from build123d import *

# Parameters (mm, degrees)
SKETCH1_W               = 40.35
SKETCH1_H               = 43.35
BOSS_EXTRUDE1_DEPTH     = 47
CUT_EXTRUDE2_DEPTH      = 102
FILLET1_R               = 10
CUT_EXTRUDE3_DEPTH      = 102
FILLET2_R               = 5
SKETCH6_R               = 1.73
CUT_EXTRUDE4_DEPTH      = 102
CUT_EXTRUDE4_DEPTH_BACK = 102
CUT_EXTRUDE5_DEPTH      = 102
SKETCH8_R               = 1.55
CUT_EXTRUDE6_DEPTH      = 102


with BuildPart() as part:
    # Sketch1 → Boss-Extrude1 (new body)
    with BuildSketch(Plane(origin=(0, 0, 0), x_dir=(1, 0, 0), z_dir=(0, 1, 0))):
        with Locations((-26.966212793, -29.108023223)):
            Rectangle(SKETCH1_W, SKETCH1_H)
    extrude(amount=BOSS_EXTRUDE1_DEPTH)

    # Sketch3 → Cut-Extrude2 (cut)
    with BuildSketch(Plane.XY.offset(50.783023223)):
        with BuildLine():
            Line((-47.141212793, 47), (-47.141212793, 26.825))
            ThreePointArc((-47.141212793, 26.825), (-41.232092103, 41.09087931), (-26.966212793, 47))
            Line((-26.966212793, 47), (-47.141212793, 47))
        make_face()
        with BuildLine():
            Line((-6.791212793, 47), (-26.966212793, 47))
            ThreePointArc((-26.966212793, 47), (-12.700333482, 41.09087931), (-6.791212793, 26.825))
            Line((-6.791212793, 26.825), (-6.791212793, 47))
        make_face()
    extrude(amount=-CUT_EXTRUDE2_DEPTH, mode=Mode.SUBTRACT)

    # Fillet1
    fillet1_edges = [part.edges().sort_by_distance(p)[0] for p in [
        (-26.966212793, 0, 50.783023223),
    ]]
    fillet(fillet1_edges, radius=FILLET1_R)

    # Sketch5 → Cut-Extrude3 (cut)
    with BuildSketch(Plane.ZY.offset(47.141212793)):
        with BuildLine():
            Line((-6.665763497, 3.45), (36.595559978, 3.45))
            Line((36.595559978, 3.45), (40.783023223, 3.45))
            ThreePointArc((40.783023223, 3.45), (45.41457264, 5.368450583), (47.333023223, 10))
            Line((47.333023223, 10), (47.333023223, 17.578484004))
            Line((47.333023223, 17.578484004), (47.333023223, 59.778436909))
            Line((47.333023223, 59.778436909), (-6.665763497, 59.778436909))
            Line((-6.665763497, 59.778436909), (-6.665763497, 3.45))
        make_face()
    extrude(amount=-CUT_EXTRUDE3_DEPTH, mode=Mode.SUBTRACT)

    # Fillet2
    fillet2_edges = [part.edges().sort_by_distance(p)[0] for p in [
        (-6.791212793, 1.725, 7.433023223),
        (-47.141212793, 1.725, 7.433023223),
    ]]
    fillet(fillet2_edges, radius=FILLET2_R)

    # Sketch6 → Cut-Extrude4 (cut, two sides)
    with BuildSketch(Plane(origin=(0, 3.45, 0), x_dir=(1, 0, 0), z_dir=(0, 1, 0))) as cut_extrude4_sk:
        with BuildLine():
            Line((-10.653989329, -40.783023223), (-13.388436256, -40.783023223))
            ThreePointArc((-13.388436256, -40.783023223), (-12.021212793, -41.453023223), (-10.653989329, -40.783023223))
        make_face()
        with BuildLine():
            ThreePointArc((-12.021212793, -37.993023223), (-13.57470885, -38.961741409), (-13.388436256, -40.783023223))
            Line((-13.388436256, -40.783023223), (-10.653989329, -40.783023223))
            ThreePointArc((-10.653989329, -40.783023223), (-10.384417663, -40.283203287), (-10.291212793, -39.723023223))
            ThreePointArc((-10.291212793, -39.723023223), (-10.797918061, -38.499728491), (-12.021212793, -37.993023223))
        make_face()
        with BuildLine():
            ThreePointArc((-41.911212793, -37.993023223), (-43.134507524, -38.499728491), (-43.641212793, -39.723023223))
            ThreePointArc((-43.641212793, -39.723023223), (-43.548007922, -40.283203287), (-43.278436256, -40.783023223))
            Line((-43.278436256, -40.783023223), (-40.543989329, -40.783023223))
            ThreePointArc((-40.543989329, -40.783023223), (-40.274417663, -40.283203287), (-40.181212793, -39.723023223))
            ThreePointArc((-40.181212793, -39.723023223), (-40.687918061, -38.499728491), (-41.911212793, -37.993023223))
        make_face()
        with BuildLine():
            Line((-40.543989329, -40.783023223), (-43.278436256, -40.783023223))
            ThreePointArc((-43.278436256, -40.783023223), (-41.911212793, -41.453023223), (-40.543989329, -40.783023223))
        make_face()
        with Locations((-12.021212793, -15.663023223)):
            Circle(SKETCH6_R)
        with Locations((-41.911212793, -15.663023223)):
            Circle(SKETCH6_R)
    extrude(amount=CUT_EXTRUDE4_DEPTH, mode=Mode.SUBTRACT)
    extrude(cut_extrude4_sk.sketch, amount=-CUT_EXTRUDE4_DEPTH_BACK, mode=Mode.SUBTRACT)

    # Sketch7 → Cut-Extrude5 (cut)
    with BuildSketch(Plane.XY.offset(50.783023223)):
        with BuildLine():
            Line((-33.541212793, 33.925), (-33.541212793, 19.945))
            ThreePointArc((-33.541212793, 19.945), (-26.966212793, 13.37), (-20.391212793, 19.945))
            Line((-20.391212793, 19.945), (-20.391212793, 33.925))
            ThreePointArc((-20.391212793, 33.925), (-26.966212793, 40.5), (-33.541212793, 33.925))
        make_face()
    extrude(amount=-CUT_EXTRUDE5_DEPTH, mode=Mode.SUBTRACT)

    # Sketch8 → Cut-Extrude6 (cut)
    with BuildSketch(Plane.XY.offset(50.783023223)):
        with Locations((-42.516212793, 26.825)):
            Circle(SKETCH8_R)
        with Locations((-34.766212793, 40.277230298)):
            Circle(SKETCH8_R)
        with Locations((-34.766212793, 13.372769702)):
            Circle(SKETCH8_R)
        with Locations((-19.166212793, 13.372769702)):
            Circle(SKETCH8_R)
        with Locations((-11.416212793, 26.825)):
            Circle(SKETCH8_R)
        with Locations((-19.166212793, 40.277230298)):
            Circle(SKETCH8_R)
    extrude(amount=-CUT_EXTRUDE6_DEPTH, mode=Mode.SUBTRACT)


solid = part.part
Build history of the part. All positions in model axes, mm. A direction names the side the tool comes from. Coordinates: 2 decimals unless noted, no trailing zeros. Order: outer loops, then holes, each group sorted by start corner. A loop starts at its lowest first (then second) coordinate and runs counter-clockwise, first axis right, second up. Notation, with made-up numbers: M 10.25,-37 L 57.25,-37 A15 ccw 57.25,-17 Z; hole C 36,77 d4. An arc over 180 degrees is marked long. One line per question, with ' | ' between items. Start each with the question number.
Q1. Saw through at A-A (y = 37). List the corners of the cut face in (x, z), then the cut area to 3 significant figures.
Q2. Two-plate mould, pull along X, no slides. Class faces 4 (the face through (-35.909, 41.325, 49.082)), 5 (the face through (-20.391, 27, 49)), 6 (the face through (-45.72, 1.75, 8.94)), 7 (the face through (-27, 3.45, 24)): +X half, -X half, draft (parallel to the pull), parting line (faces both ways), or undercut.
Q3. Saw through at C-C (y = 14). List the corners of the cut face in (x, z), then the cut area to 3 significant figures.
Q4. Saw through at D-D (x = -18.5). List the corners of the cut face in (y, z), then the cut area to 3 significant figures.
Q5. Saw through at B-B (x = -26). List the corners of the cut face in (y, z), then the cut area to 3 significant figures.
Q6. Flat gauge pins, fed straight in: pin 1 Ø2.5 at (x, y) = (-19.17, 40.28) entering from -Z; pin 2 Ø4 at (x, z) = (-12.02, 15.66) entering from +Y; pin 3 Ø2 at (x, y) = (-30.5, 15) entering from -Z. Where does each tip first touch, or does it go through?
Q7. 3-axis set-ups, long thin cutter, end or side, ignore diameter. For faces 1 (the face through (-26.82, 40.5, 49.08)), 2 (the face through (-18, 28, 47.333)), 3 (the face through (-27, 2, 7.433)): which of +Z, -Z, +X, -X, +Y, -Y reach the whole face in a straight line?
Q8. Probe L1, parallel to X at y = 21.5, z = 48.5; L2, parallel to Z at x = -27.5, y = 42; L3, parallel to Y at x = -15, z = 37. List the from-to ranges inside material, lowest first. Write a range as from..to.
Check values:
1) outline: M -44.39,47.33 L -32.78,47.33 L -32.78,50.78 L -44.39,50.78 Z; M -21.15,47.33 L -9.54,47.33 L -9.54,50.78 L -21.15,50.78 Z | area: 80.1 mm2
2) face 4: undercut | face 5: undercut | face 6: -X half | face 7: draft
3) outline: M -47.14,47.33 L -36.18,47.33 L -36.18,50.78 L -47.14,50.78 Z; M -33.35,47.33 L -29.77,47.33 L -29.77,50.78 L -33.35,50.78 Z; M -24.16,47.33 L -20.58,47.33 L -20.58,50.78 L -24.16,50.78 Z; M -17.75,47.33 L -6.79,47.33 L -6.79,50.78 L -17.75,50.78 Z | area: 100 mm2
4) outline: M 0,7.43 L 3.45,7.43 L 3.45,40.78 A6.55 cw 10,47.33 L 11.97,47.33 L 11.97,50.78 L 10,50.78 A10 ccw 0,40.78 Z; M 14.77,47.33 L 38.88,47.33 L 38.88,50.78 L 14.77,50.78 Z; M 41.68,47.33 L 45.14,47.33 L 45.14,50.78 L 41.68,50.78 Z | area: 262 mm2
5) outline: M 0,7.43 L 3.45,7.43 L 3.45,40.78 A6.55 cw 10,47.33 L 13.44,47.33 L 13.44,50.78 L 10,50.78 A10 ccw 0,40.78 Z; M 40.43,47.33 L 46.98,47.33 L 46.98,50.78 L 40.43,50.78 Z | area: 194 mm2
6) pin 1: passes through | pin 2: stops at y = 3.45 | pin 3: stops at z = 47.33
7) face 1: +Z, -Z | face 2: -Z, +X, -X, +Y | face 3: -Z, +X, -X, +Y, -Y
8) L1: x = -47.14..-33.54, -20.39..-6.79 | L2: z = 47.33..50.78 | L3: y = 0..3.45
